Can you work these out from the model? Positions are in its coordinate system, mm. A direction names the side the tool comes from. Give positions to 0.01 mm unless a question says otherwise; leave off trailing zeros. Write each loop counter-clockwise with the first axis right and the second up, starting at its lowest first coordinate (ties: lowest second). Pieces come first, ordered by that corner, then holes. Notation, with made-up numbers: M 60.25,75 L 94.25,75 A18 cw 94.25,93 Z; hole C 35.5,-12.75 d7. An arc over 180 degrees is marked long. Use CSV: the item, a comma, the result in double quotes. Start each with the question number.
from build123d import *

# Parameters (mm, degrees)
F0_W     = 101.6
F0_H     = 76.2
F0_R     = 1.27
F0_W_2   = 88.9
F0_H_2   = 44.45
F1_DEPTH = 3.175


with BuildPart() as f1:
    # F0 (on Right) → F1 (new body)
    with BuildSketch(Plane.YZ):
        Rectangle(F0_W, F0_H)
        with Locations((-39.243757, -25.4)):
            Circle(F0_R, mode=Mode.SUBTRACT)
        with Locations((-32.893757, -25.4)):
            Circle(F0_R, mode=Mode.SUBTRACT)
        with Locations((-26.543757, -25.4)):
            Circle(F0_R, mode=Mode.SUBTRACT)
        with Locations((-20.193757, -25.4)):
            Circle(F0_R, mode=Mode.SUBTRACT)
        with Locations((-13.843757, -25.4)):
            Circle(F0_R, mode=Mode.SUBTRACT)
        with Locations((-7.493757, -25.4)):
            Circle(F0_R, mode=Mode.SUBTRACT)
        with Locations((-1.143757, -25.4)):
            Circle(F0_R, mode=Mode.SUBTRACT)
        with Locations((5.206243, -25.4)):
            Circle(F0_R, mode=Mode.SUBTRACT)
        with Locations((11.556243, -25.4)):
            Circle(F0_R, mode=Mode.SUBTRACT)
        with Locations((17.906243, -25.4)):
            Circle(F0_R, mode=Mode.SUBTRACT)
        with Locations((24.256243, -25.4)):
            Circle(F0_R, mode=Mode.SUBTRACT)
        with Locations((30.606243, -25.4)):
            Circle(F0_R, mode=Mode.SUBTRACT)
        with Locations((36.956243, -25.4)):
            Circle(F0_R, mode=Mode.SUBTRACT)
        with Locations((0, 9.525)):
            Rectangle(F0_W_2, F0_H_2, mode=Mode.SUBTRACT)
    extrude(amount=F1_DEPTH)


solid = f1.part
(1) I want a section at A-A (z = -1.5). Write out the boundary of the cut face in (x, y) (3 decimals), and give its area (3 significant figures).
(2) I want a section at C-C (x = 0.95). State how many separate pieces and enclosed holes the cut face has, and give its area (3 significant figures).
(3) I want a section at B-B (y = 27.5). Write out the boundary of the cut face in (x, z) (3 decimals), and give its area (3 significant figures).
(4) Thinking about a two-plate mould opening in Z: for faces 3 (the face through (2, -1, 38.1)), 4 (the face through (3.175, -12, -16)), 5 (the face through (1.57, -31.68, -25.02)), which applies, released by +Z, released by -Z, zero draft, split by the parting line, or undercut?
(5) Will this pin go through, and if not, where does the flat tip stop? pin 1 Ø1.5 at (y, z) = (24.26, -25.4) entering from +X.
(6) Please list where these lines run through material, in increasing order: L1, parallel to Z at x = 1.1, y = -39; L2, parallel to Z at x = 2.45, y = 30.5; L3, parallel to Z at x = 2, y = 39.5. Write a range as [from, to].
(7) Which directions (+Z, -Z, +X, -X, +Y, -Y) give clear straight access to the entire face, cutting with the end or side of a thin tool? Please do faces 1 (the face through (2, -1, 31.75)), 2 (the face through (0, -12, -16)).
Geometry results:
1,outline,"M 0,-50.8 L 3.175,-50.8 L 3.175,-44.45 L 0,-44.45 Z; M 0,44.45 L 3.175,44.45 L 3.175,50.8 L 0,50.8 Z"
1,area,"40.3 mm2"
2,separate pieces,"1"
2,enclosed holes,"14"
2,area,"3,720 mm2"
3,outline,"M 0,-38.1 L 3.175,-38.1 L 3.175,-12.7 L 0,-12.7 Z; M 0,31.75 L 3.175,31.75 L 3.175,38.1 L 0,38.1 Z"
3,area,"101 mm2"
4,face 3,"released by +Z"
4,face 4,"zero draft"
4,face 5,"undercut"
5,pin 1,"passes through"
6,L1,"z = [-38.1, -26.65], [-24.15, -12.7], [31.75, 38.1]"
6,L2,"z = [-38.1, -26.67], [-24.13, -12.7], [31.75, 38.1]"
6,L3,"z = [-38.1, -12.7], [31.75, 38.1]"
7,face 1,"+X, -X"
7,face 2,"+Z, -Z, -X, +Y, -Y"
